```python
from build123d import *

# Parameters (mm, degrees)
SKETCH2_R           = 18.85
BOSS_EXTRUDE1_DEPTH = 5


with BuildPart() as part:
    # Sketch2 → Boss-Extrude1 (new body)
    with BuildSketch(Plane.XY.offset(10)):
        Circle(SKETCH2_R)
        with BuildLine():
            Line((-6.800750564, 11.632097199), (-6.80194974, 8.632097439))
            ThreePointArc((-6.80194974, 8.632097439), (-7.802349385, 7.632497244), (-8.80194958, 8.632896889))
            Line((-8.80194958, 8.632896889), (-8.800750404, 11.63289665))
            ThreePointArc((-8.800750404, 11.63289665), (-7.800350759, 12.632496845), (-6.800750564, 11.632097199))
        make_face(mode=Mode.SUBTRACT)
        with BuildLine():
            Line((-4.900750404, 11.63289665), (-4.90194958, 8.632896889))
            ThreePointArc((-4.90194958, 8.632896889), (-3.902349385, 7.632497244), (-2.90194974, 8.632097439))
            Line((-2.90194974, 8.632097439), (-2.900750564, 11.632097199))
            ThreePointArc((-2.900750564, 11.632097199), (-3.900350759, 12.632496845), (-4.900750404, 11.63289665))
        make_face(mode=Mode.SUBTRACT)
        with BuildLine():
            Line((-1.000750404, 11.63289665), (-1.00194958, 8.632896889))
            ThreePointArc((-1.00194958, 8.632896889), (-0.002349385, 7.632497244), (0.99805026, 8.632097439))
            Line((0.99805026, 8.632097439), (0.999249436, 11.632097199))
            ThreePointArc((0.999249436, 11.632097199), (-0.000350759, 12.632496845), (-1.000750404, 11.63289665))
        make_face(mode=Mode.SUBTRACT)
        with BuildLine():
            Line((2.899249596, 11.63289665), (2.89805042, 8.632896889))
            ThreePointArc((2.89805042, 8.632896889), (3.897650615, 7.632497244), (4.89805026, 8.632097439))
            Line((4.89805026, 8.632097439), (4.899249436, 11.632097199))
            ThreePointArc((4.899249436, 11.632097199), (3.899649241, 12.632496845), (2.899249596, 11.63289665))
        make_face(mode=Mode.SUBTRACT)
        with BuildLine():
            Line((6.799249596, 11.63289665), (6.79805042, 8.632896889))
            ThreePointArc((6.79805042, 8.632896889), (7.797650615, 7.632497244), (8.79805026, 8.632097439))
            Line((8.79805026, 8.632097439), (8.799249436, 11.632097199))
            ThreePointArc((8.799249436, 11.632097199), (7.799649241, 12.632496845), (6.799249596, 11.63289665))
        make_face(mode=Mode.SUBTRACT)
        with BuildLine():
            Line((-10.703450753, 1.876998531), (-10.7019502, 4.876998531))
            ThreePointArc((-10.7019502, 4.876998531), (-11.701449891, 5.87749859), (-12.70194995, 4.877998899))
            Line((-12.70194995, 4.877998899), (-12.703450502, 1.877998899))
            ThreePointArc((-12.703450502, 1.877998899), (-11.703950811, 0.87749884), (-10.703450753, 1.876998531))
        make_face(mode=Mode.SUBTRACT)
        with BuildLine():
            Line((-8.803450087, 1.877998899), (-8.801949535, 4.877998899))
            ThreePointArc((-8.801949535, 4.877998899), (-7.801449476, 5.87749859), (-6.801949785, 4.876998531))
            Line((-6.801949785, 4.876998531), (-6.803450337, 1.876998531))
            ThreePointArc((-6.803450337, 1.876998531), (-7.803950396, 0.87749884), (-8.803450087, 1.877998899))
        make_face(mode=Mode.SUBTRACT)
        with BuildLine():
            Line((-2.903450337, 1.876998531), (-2.901949785, 4.876998531))
            ThreePointArc((-2.901949785, 4.876998531), (-3.901449476, 5.87749859), (-4.901949535, 4.877998899))
            Line((-4.901949535, 4.877998899), (-4.903450087, 1.877998899))
            ThreePointArc((-4.903450087, 1.877998899), (-3.903950396, 0.87749884), (-2.903450337, 1.876998531))
        make_face(mode=Mode.SUBTRACT)
        with BuildLine():
            Line((0.996549663, 1.876998531), (0.998050215, 4.876998531))
            ThreePointArc((0.998050215, 4.876998531), (-0.001449476, 5.87749859), (-1.001949535, 4.877998899))
            Line((-1.001949535, 4.877998899), (-1.003450087, 1.877998899))
            ThreePointArc((-1.003450087, 1.877998899), (-0.003950396, 0.87749884), (0.996549663, 1.876998531))
        make_face(mode=Mode.SUBTRACT)
        with BuildLine():
            Line((4.896549663, 1.876998531), (4.898050215, 4.876998531))
            ThreePointArc((4.898050215, 4.876998531), (3.898550524, 5.87749859), (2.898050465, 4.877998899))
            Line((2.898050465, 4.877998899), (2.896549913, 1.877998899))
            ThreePointArc((2.896549913, 1.877998899), (3.896049604, 0.87749884), (4.896549663, 1.876998531))
        make_face(mode=Mode.SUBTRACT)
        with BuildLine():
            Line((8.796549663, 1.876998531), (8.798050215, 4.876998531))
            ThreePointArc((8.798050215, 4.876998531), (7.798550524, 5.87749859), (6.798050465, 4.877998899))
            Line((6.798050465, 4.877998899), (6.796549913, 1.877998899))
            ThreePointArc((6.796549913, 1.877998899), (7.796049604, 0.87749884), (8.796549663, 1.876998531))
        make_face(mode=Mode.SUBTRACT)
        with BuildLine():
            Line((12.696549663, 1.876998531), (12.698050215, 4.876998531))
            ThreePointArc((12.698050215, 4.876998531), (11.698550524, 5.87749859), (10.698050465, 4.877998899))
            Line((10.698050465, 4.877998899), (10.696549913, 1.877998899))
            ThreePointArc((10.696549913, 1.877998899), (11.696049604, 0.87749884), (12.696549663, 1.876998531))
        make_face(mode=Mode.SUBTRACT)
        with BuildLine():
            Line((-8.804648151, -4.877758991), (-8.800750032, -1.877758991))
            ThreePointArc((-8.800750032, -1.877758991), (-7.799451504, -0.879059207), (-6.80075172, -1.880357735))
            Line((-6.80075172, -1.880357735), (-6.80464984, -4.880357735))
            ThreePointArc((-6.80464984, -4.880357735), (-7.805948368, -5.879057519), (-8.804648151, -4.877758991))
        make_face(mode=Mode.SUBTRACT)
        with BuildLine():
            Line((-2.90464984, -4.880357735), (-2.90075172, -1.880357735))
            ThreePointArc((-2.90075172, -1.880357735), (-3.899451504, -0.879059207), (-4.900750032, -1.877758991))
            Line((-4.900750032, -1.877758991), (-4.904648151, -4.877758991))
            ThreePointArc((-4.904648151, -4.877758991), (-3.905948368, -5.879057519), (-2.90464984, -4.880357735))
        make_face(mode=Mode.SUBTRACT)
        with BuildLine():
            Line((0.99535016, -4.880357735), (0.99924828, -1.880357735))
            ThreePointArc((0.99924828, -1.880357735), (0.000548496, -0.879059207), (-1.000750032, -1.877758991))
            Line((-1.000750032, -1.877758991), (-1.004648151, -4.877758991))
            ThreePointArc((-1.004648151, -4.877758991), (-0.005948368, -5.879057519), (0.99535016, -4.880357735))
        make_face(mode=Mode.SUBTRACT)
        with BuildLine():
            Line((4.89535016, -4.880357735), (4.89924828, -1.880357735))
            ThreePointArc((4.89924828, -1.880357735), (3.900548496, -0.879059207), (2.899249968, -1.877758991))
            Line((2.899249968, -1.877758991), (2.895351849, -4.877758991))
            ThreePointArc((2.895351849, -4.877758991), (3.894051632, -5.879057519), (4.89535016, -4.880357735))
        make_face(mode=Mode.SUBTRACT)
        with BuildLine():
            Line((8.79535016, -4.880357735), (8.79924828, -1.880357735))
            ThreePointArc((8.79924828, -1.880357735), (7.800548496, -0.879059207), (6.799249968, -1.877758991))
            Line((6.799249968, -1.877758991), (6.795351849, -4.877758991))
            ThreePointArc((6.795351849, -4.877758991), (7.794051632, -5.879057519), (8.79535016, -4.880357735))
        make_face(mode=Mode.SUBTRACT)
        with BuildLine():
            Line((12.69535016, -4.880357735), (12.69924828, -1.880357735))
            ThreePointArc((12.69924828, -1.880357735), (11.700548496, -0.879059207), (10.699249968, -1.877758991))
            Line((10.699249968, -1.877758991), (10.695351849, -4.877758991))
            ThreePointArc((10.695351849, -4.877758991), (11.694051632, -5.879057519), (12.69535016, -4.880357735))
        make_face(mode=Mode.SUBTRACT)
        with BuildLine():
            Line((-10.70464984, -4.880357735), (-10.70075172, -1.880357735))
            ThreePointArc((-10.70075172, -1.880357735), (-11.699451504, -0.879059207), (-12.700750032, -1.877758991))
            Line((-12.700750032, -1.877758991), (-12.704648151, -4.877758991))
            ThreePointArc((-12.704648151, -4.877758991), (-11.705948368, -5.879057519), (-10.70464984, -4.880357735))
        make_face(mode=Mode.SUBTRACT)
        with BuildLine():
            Line((-6.800749353, -8.635615621), (-6.800749353, -11.635615621))
            ThreePointArc((-6.800749353, -11.635615621), (-7.800749353, -12.635615621), (-8.800749353, -11.635615621))
            Line((-8.800749353, -11.635615621), (-8.800749353, -8.635615621))
            ThreePointArc((-8.800749353, -8.635615621), (-7.800749353, -7.635615621), (-6.800749353, -8.635615621))
        make_face(mode=Mode.SUBTRACT)
        with BuildLine():
            Line((-4.900749353, -8.635615621), (-4.900749353, -11.635615621))
            ThreePointArc((-4.900749353, -11.635615621), (-3.900749353, -12.635615621), (-2.900749353, -11.635615621))
            Line((-2.900749353, -11.635615621), (-2.900749353, -8.635615621))
            ThreePointArc((-2.900749353, -8.635615621), (-3.900749353, -7.635615621), (-4.900749353, -8.635615621))
        make_face(mode=Mode.SUBTRACT)
        with BuildLine():
            Line((-1.000749353, -8.635615621), (-1.000749353, -11.635615621))
            ThreePointArc((-1.000749353, -11.635615621), (-0.000749353, -12.635615621), (0.999250647, -11.635615621))
            Line((0.999250647, -11.635615621), (0.999250647, -8.635615621))
            ThreePointArc((0.999250647, -8.635615621), (-0.000749353, -7.635615621), (-1.000749353, -8.635615621))
        make_face(mode=Mode.SUBTRACT)
        with BuildLine():
            Line((2.899250647, -8.635615621), (2.899250647, -11.635615621))
            ThreePointArc((2.899250647, -11.635615621), (3.899250647, -12.635615621), (4.899250647, -11.635615621))
            Line((4.899250647, -11.635615621), (4.899250647, -8.635615621))
            ThreePointArc((4.899250647, -8.635615621), (3.899250647, -7.635615621), (2.899250647, -8.635615621))
        make_face(mode=Mode.SUBTRACT)
        with BuildLine():
            Line((6.799250647, -8.635615621), (6.799250647, -11.635615621))
            ThreePointArc((6.799250647, -11.635615621), (7.799250647, -12.635615621), (8.799250647, -11.635615621))
            Line((8.799250647, -11.635615621), (8.799250647, -8.635615621))
            ThreePointArc((8.799250647, -8.635615621), (7.799250647, -7.635615621), (6.799250647, -8.635615621))
        make_face(mode=Mode.SUBTRACT)
    extrude(amount=BOSS_EXTRUDE1_DEPTH)


solid = part.part
```
Geometry check sheet. Reference: the model listing, model coordinates, mm. A direction names the side the tool comes from. Round coordinates to 2 decimals unless told otherwise and drop trailing zeros. Write each loop counter-clockwise with the first axis right and the second up, starting at its lowest first coordinate (ties: lowest second). Pieces come first, ordered by that corner, then holes. Notation, with made-up numbers: (24, 26) - (55, 26) arc R20 cw to (55, 41) - close; hole circle Ø1 at (-22.75, 33). An arc over 180 degrees is marked (long way). Write each question's results on one line, items separated by ' | '.
(1) Depth check by flat-ended pin: pin 1 Ø2.5 at (y, z) = (10, 13) entering from -X; pin 2 Ø0.9 at (y, z) = (9.5, 13) entering from +X; pin 3 Ø0.9 at (y, z) = (-11, 11.5) entering from -X. Enter the tip coordinate at first touch or a pass-through.
Computed:
pin 1: stops at x = -16.7 | pin 2: stops at x = 16.54 | pin 3: stops at x = -15.62
(2) Sectioned sample at D-D, the plane y = -15. Enter the section's corners in (x, z).
Computed:
outline: (-11.42, 10) - (11.42, 10) - (11.42, 15) - (-11.42, 15) - close
(3) Sectioned sample at A-A, the plane x = 0. Enter the section's corners in (y, z), plus the area to 3 significant figures.
Computed:
outline: (-18.85, 10) - (-12.64, 10) - (-12.64, 15) - (-18.85, 15) - close; (-7.64, 10) - (-5.88, 10) - (-5.88, 15) - (-7.64, 15) - close; (-0.88, 10) - (0.88, 10) - (0.88, 15) - (-0.88, 15) - close; (5.88, 10) - (7.63, 10) - (7.63, 15) - (5.88, 15) - close; (12.63, 10) - (18.85, 10) - (18.85, 15) - (12.63, 15) - close | area: 88.5 mm^2
(4) Thickness scan on probe 1 along X at (y, z) = (12, 12.6); probe 2 along Y at (x, z) = (11, 12.5); probe 3 along Y at (x, z) = (-3, 12.3). Record the ranges inside material, lowest first. Write a range as from..to.
Computed:
probe 1: x = -14.54..-8.73, -6.87..-4.83, -2.97..-0.93, 0.93..2.97, 4.83..6.87, 8.73..14.54 | probe 2: y = -15.31..-5.6, -1.16..1.16, 5.59..15.31 | probe 3: y = -18.61..-12.07, -8.2..-5.31, -1.44..1.45, 5.31..8.2, 12.07..18.61
(5) Draft check along Y on faces 1 (the face through (-0.026, 0.878, 12.465)), 2 (the face through (0, 0, 10)). Enter one of: pulls with the +Y half, pulls with the -Y half, needs draft (parallel to the pull), parting line crosses it, or undercut.
Computed:
face 1: undercut | face 2: needs draft
(6) Sectioned sample at B-B, the plane z = 12.1. Count the separate pieces of the cut face and the enclosed holes in it, plus the area to 3 significant figures.
Computed:
separate pieces: 1 | enclosed holes: 24 | area: 897 mm^2
(7) Set-up check for faces 3 (the face through (-7.823, -7.636, 12.465)), 4 (the face through (0, 0, 15)): record each of +Z, -Z, +X, -X, +Y, -Y from which the full face is reachable in a straight line by a thin tool's end or side.
Computed:
face 3: +Z, -Z | face 4: +Z, +X, -X, +Y, -Y
(8) Sectioned sample at C-C, the plane x = 10. Enter the section's corners in (y, z), plus the area to 3 significant figures.
Computed:
outline: (-15.98, 10) - (15.98, 10) - (15.98, 15) - (-15.98, 15) - close | area: 160 mm^2
